Here's how the part is built. I have some questions about the finished solid (model axes, mm). Round coordinates to 2 decimals unless told otherwise and drop trailing zeros. Order: outer loops, then holes, each group sorted by start corner. A loop starts at its lowest first (then second) coordinate and runs counter-clockwise, first axis right, second up.
```python
from build123d import *

# Parameters (mm, degrees)
SKETCH2_R                       = 4.995
BOSS_EXTRUDE1_DEPTH             = 119
F_5_0MM_DOWEL_HOLE1_D           = 5
F_5_0MM_DOWEL_HOLE1_CSINK_D     = 5.05
F_5_0MM_DOWEL_HOLE1_CSINK_ANGLE = 90
F_5_0MM_DOWEL_HOLE2_D           = 5
F_5_0MM_DOWEL_HOLE2_CSINK_D     = 5.05
F_5_0MM_DOWEL_HOLE2_CSINK_ANGLE = 90


with BuildPart() as part:
    # Sketch2 → Boss-Extrude1 (new body)
    with BuildSketch(Plane.XY):
        Circle(SKETCH2_R)
    extrude(amount=BOSS_EXTRUDE1_DEPTH)

    # Ø5.0mm Dowel Hole1 (through all)
    with Locations(Plane.ZY.offset(4.995)):
        with Locations((13, 0)):
            f_5_0mm_dowel_hole1 = CounterSinkHole(F_5_0MM_DOWEL_HOLE1_D / 2, F_5_0MM_DOWEL_HOLE1_CSINK_D / 2, counter_sink_angle=F_5_0MM_DOWEL_HOLE1_CSINK_ANGLE)

    # Mirror1: Ø5.0mm Dowel Hole1 across plane
    add(f_5_0mm_dowel_hole1.mirror(Plane(origin=(0, 0, 59.5), x_dir=(1, 0, 0), z_dir=(0, 0, -1))), mode=Mode.SUBTRACT)

    # Ø5.0mm Dowel Hole2 (through all)
    with Locations(Plane.ZY.offset(4.995)):
        with Locations((86.98, 0)):
            CounterSinkHole(F_5_0MM_DOWEL_HOLE2_D / 2, F_5_0MM_DOWEL_HOLE2_CSINK_D / 2, counter_sink_angle=F_5_0MM_DOWEL_HOLE2_CSINK_ANGLE)


solid = part.part
```
1) If we section it at A-A (x = 0): Write out the boundary of the cut face in (y, z) (3 decimals).
2) I need wall thicknesses on line 1 (Z direction, x = 1.75, y = 0); line 2 (Z direction, x = 3, y = -0.5); line 3 (Y direction, x = 0.25, z = 86.98). Which ranges of each line are inside material? Lowest first, please.
3) I'm going to push flat-ended pins straight in: pin 1 (1.5 mm diameter, centred on y = -3, z = 25.5, fed in from -X); pin 2 (5 mm diameter, centred on x = 3.5, z = 19, fed in from +Y); pin 3 (4.5 mm diameter, centred on y = 0, z = 106, fed in from +X); pin 4 (1 mm diameter, centred on y = 1.5, z = 29, fed in from -X). Where does each tip first touch, or does it pass through?
4) If we section it at C-C (z = 102): Write out the boundary of the cut face in (x, y) (3 decimals), plus the area to 3 significant figures.
5) If we section it at D-D (z = 86.98): Write out the boundary of the cut face in (x, y) (3 decimals).
6) We'd pull the mould along Z, two halves only. Please class faces 1 (the flat face through (0, 0, 0)), 2 (the flat face through (0, 0, 119)), 3 (the cylindrical face through (0.08, -2.22, 85.83)): +Z half, -Z half, draft (parallel to the pull), parting line (faces both ways), or undercut.
7) If we section it at B-B (y = -1.5): Write out the boundary of the cut face in (x, z), plus the area to 3 significant figures.
Solutions:
1. outline: (-4.995, 0) - (4.995, 0) - (4.995, 119) - (-4.995, 119) - close; hole circle Ø5 at (0, 13); hole circle Ø5 at (0, 86.98); hole circle Ø5 at (0, 106)
2. line 1: z = 0 to 10.5, 15.5 to 84.48, 89.48 to 103.5, 108.5 to 119
2. line 2: z = 0 to 10.55, 15.45 to 84.53, 89.43 to 103.55, 108.45 to 119
2. line 3: y = -4.99 to -2.5, 2.5 to 4.99
3. pin 1: stops at x = -4.46
3. pin 2: stops at y = 4.89
3. pin 3: passes through
3. pin 4: stops at x = -4.89
4. outline: circle Ø9.99 at (0, 0)
4. area: 78.4 mm2
5. outline: (-4.324, -2.5) arc R4.995 ccw to (4.324, -2.5) - close; (-4.324, 2.5) - (4.324, 2.5) arc R4.995 ccw to start
6. face 1: -Z half
6. face 2: +Z half
6. face 3: undercut
7. outline: (-4.76, 0) - (4.76, 0) - (4.76, 11) - (-4.76, 11) - close; (-4.76, 15) - (4.76, 15) - (4.76, 84.98) - (-4.76, 84.98) - close; (-4.76, 88.98) - (4.76, 88.98) - (4.76, 104) - (-4.76, 104) - close; (-4.76, 108) - (4.76, 108) - (4.76, 119) - (-4.76, 119) - close
7. area: 1,020 mm2
